from build123d import *

# Parameters (mm, degrees)
SKETCH_1_R          = 1.984
EXTRUDE_1_DEPTH     = 6.35
SKETCH_2_W          = 6.35
SKETCH_2_H          = 28
EXTRUDE_2_DEPTH     = 60
CUT_EXTRUDE_1_DEPTH = 250


with BuildPart() as part:
    # 草图1 → 凸台-拉伸1 (new body)
    with BuildSketch(Plane(origin=(0, 0, 0), x_dir=(1, 0, 0), z_dir=(0, 1, 0))):
        Polygon((98.023064942, -74.926838383), (91.673064942, -74.926838383), (80.206659609, -74.926838383), (63.904311177, -28.766838383), (-64.490991959, -28.766838383), (-80.793340391, -74.926838383), (-92.259745724, -74.926838383), (-98.609745724, -74.926838383), (-98.609745724, 45.393161617), (-92.259745724, 45.393161617), (-80.793340391, -0.766838383), (-64.490991959, -0.766838383), (63.904311177, -0.766838383), (80.206659609, -0.766838383), (91.673064942, 45.393161617), (98.023064942, 45.393161617), align=None)
        with Locations((91.673064942, -62.226838383)):
            Circle(SKETCH_1_R, mode=Mode.SUBTRACT)
        with Locations((91.673064942, 32.693161617)):
            Circle(SKETCH_1_R, mode=Mode.SUBTRACT)
        with Locations((-92.259745724, -62.226838383)):
            Circle(SKETCH_1_R, mode=Mode.SUBTRACT)
        with Locations((-92.259745724, 32.693161617)):
            Circle(SKETCH_1_R, mode=Mode.SUBTRACT)
    extrude(amount=EXTRUDE_1_DEPTH)

    # 草图2 → 凸台-拉伸2 (add)
    with BuildSketch(Plane(origin=(0, 6.35, 0), x_dir=(1, 0, 0), z_dir=(0, 1, 0))):
        with Locations((-84.468340391, -14.766838383)):
            Rectangle(SKETCH_2_W, SKETCH_2_H)
        with Locations((83.881659609, -14.766838383)):
            Rectangle(SKETCH_2_W, SKETCH_2_H)
    extrude(amount=EXTRUDE_2_DEPTH)

    # 草图3 → 切除-拉伸1 (cut)
    with BuildSketch(Plane(origin=(87.056659609, 0, 0), x_dir=(0, 0, -1), z_dir=(1, 0, 0))):
        Polygon((-22.436838383, 62.44), (-22.436838383, 59.94), (-26.436838383, 59.94), (-26.436838383, 64.94), (-22.436838383, 64.94), align=None)
        Polygon((-16.616838383, 62.44), (-16.616838383, 59.94), (-12.616838383, 59.94), (-12.616838383, 64.94), (-16.616838383, 64.94), align=None)
        Polygon((-6.796838383, 62.44), (-6.796838383, 64.94), (-2.796838383, 64.94), (-2.796838383, 59.94), (-6.796838383, 59.94), align=None)
    extrude(amount=-CUT_EXTRUDE_1_DEPTH, mode=Mode.SUBTRACT)


solid = part.part
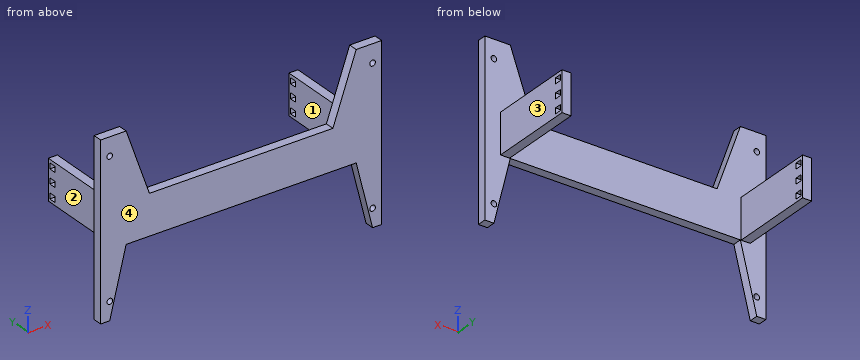
Design review of the part built by this model. Coordinates are the model's own, in mm. Face numbers are marked on the shaded views. Give positions to 0.01 mm unless a question says otherwise; leave off trailing zeros. Loops run counter-clockwise (first coordinate to the right, second up) from the corner with the lowest first, then second, coordinate; pieces in that order, holes last. Notation, with made-up numbers: (18.5, 25) - (51.5, 25) arc R15 ccw to (51.5, 54) - close; hole circle Ø3 at (-38.5, -29.5). An arc over 180 degrees is marked (long way). Write item = value, one per line.
1) Clearance check with flat-ended pins moving along their axes: pin 1 Ø5 at (x, y) = (83.5, 38.5) entering from +Z; pin 2 Ø2.5 at (x, y) = (-85.5, 63.5) entering from -Z; pin 3 Ø4 at (x, z) = (-78, 59.5) entering from +Y; pin 4 Ø3 at (x, z) = (-25.5, 4.5) entering from -Y. State where each tip first meets the part, or that it passes through.
Result sheet:
pin_1 = 28.77
pin_2 = 0.77
pin_3 = 6.35
pin_4 = 0
2) Take a section at A-A on y = 62. Count the separate pieces of the cut face and the enclosed holes in it, and give its area (3 significant figures).
Result sheet:
separate_pieces = 8
enclosed_holes = 0
area = 203 mm2
3) Take a section at C-C on x = -60. State the section outline as (y, z) points.
Result sheet:
outline = (0, 0.77) - (6.35, 0.77) - (6.35, 28.77) - (0, 28.77) - close
4) Take a section at D-D on z = 40.5. State the section outline as (x, y) points, and give its area (3 significant figures).
Result sheet:
outline = (-98.61, 0) - (-68.63, 0) - (-68.63, 6.35) - (-98.61, 6.35) - close; (68.05, 0) - (98.02, 0) - (98.02, 6.35) - (68.05, 6.35) - close
area = 381 mm2
5) Take a section at B-B on z = 58. State the section outline as (x, y) points.
Result sheet:
outline = (-98.61, 0) - (-74.82, 0) - (-74.82, 6.35) - (-98.61, 6.35) - close; (74.23, 0) - (98.02, 0) - (98.02, 6.35) - (74.23, 6.35) - close
6) To check wall thickness, follow line 1 (X direction, y = 52.5, z = 4.5); line 2 (Y direction, x = -83, z = 40.5); line 3 (Z direction, x = -82, y = 47.5). State the ranges of each line that lie inside material, in increasing order.
Result sheet:
line_1 = -87.64 to -81.29, 80.71 to 87.06
line_2 = 0 to 6.35
line_3 = 0.77 to 28.77
7) Draft analysis for pull direction X (two halves, no side actions). For the marked faces 1, 2, 3 and 4, state which applies: +X half, -X half, draft (parallel to the pull), parting line (faces both ways), or undercut.
Result sheet:
face_1 = undercut
face_2 = -X half
face_3 = +X half
face_4 = draft
